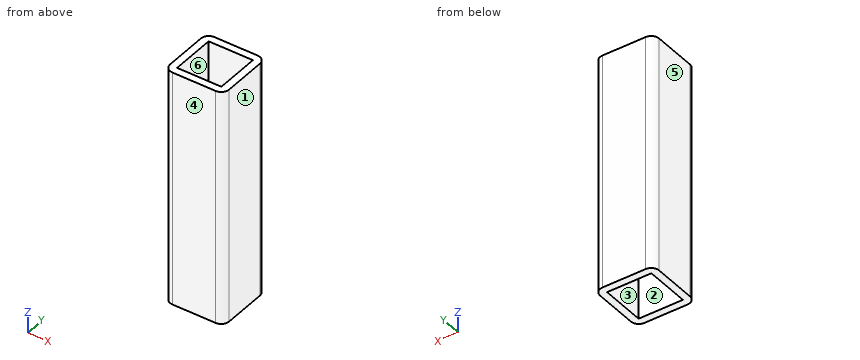
```python
from build123d import *

# Parameters (mm, degrees)
F0_W     = 38.1
F0_H     = 38.1
F0_W_2   = 28.575
F0_H_2   = 28.575
F1_DEPTH = 152.4
F2_R     = 5.08


with BuildPart() as f1:
    # F0 (on Top) → F1 (new body)
    with BuildSketch(Plane.XY):
        Rectangle(F0_W, F0_H)
        Rectangle(F0_W_2, F0_H_2, mode=Mode.SUBTRACT)
    extrude(amount=-F1_DEPTH)

    # F2
    f2_edges = [f1.edges().sort_by_distance(p)[0] for p in [
        (19.05, -19.05, -76.2),
        (19.05, 19.05, -76.2),
        (-19.05, -19.05, -76.2),
        (-19.05, 19.05, -76.2),
    ]]
    fillet(f2_edges, radius=F2_R)


solid = f1.part
```
Geometry check sheet. Reference: the model listing, model coordinates, mm. Face numbers are marked on the shaded views. A direction names the side the tool comes from. Round coordinates to 2 decimals unless told otherwise and drop trailing zeros. Order: outer loops, then holes, each group sorted by start corner. A loop starts at its lowest first (then second) coordinate and runs counter-clockwise, first axis right, second up. Notation, with made-up numbers: (19, 87.25) - (42, 87.25) arc R12 cw to (42, 103.25) - close; hole circle Ø10 at (-27.75, 86.25). An arc over 180 degrees is marked (long way). Use a Markdown table: item, result. Add a question column.
(1) Release check for a two-part mould opening along Y. For the marked faces 1, 2, 3 and 4 record: pulls with the +Y half, pulls with the -Y half, needs draft (parallel to the pull), parting line crosses it, or undercut.
(2) Material ranges on line 1 along X through (y, z) = (3.5, -39); line 2 along X through (y, z) = (14.5, -125.5), recorded low to high. Write a range as [from, to].
(3) Tool access check on the marked faces 5 and 6. Record the directions out of +Z, -Z, +X, -X, +Y, -Y that give a thin tool (end or side, any length) a straight path to the whole face; none if there is none.
(4) Sectioned sample at A-A, the plane x = -10. Enter the section's corners in (y, z).
(5) Sectioned sample at B-B, the plane z = -139.5. Enter the section's corners in (x, y), and give its area (3 significant figures).
Answers below:
| question | item | result |
|---|---|---|
| 1 | face 1 | needs draft |
| 1 | face 2 | undercut |
| 1 | face 3 | undercut |
| 1 | face 4 | pulls with the -Y half |
| 2 | line 1 | [-19.05, -14.29], [14.29, 19.05] |
| 2 | line 2 | [-19.02, 19.02] |
| 3 | face 5 | +Z, -Z, -X, +Y, -Y |
| 3 | face 6 | +Z, -Z |
| 4 | outline | (-19.05, -152.4) - (-14.29, -152.4) - (-14.29, 0) - (-19.05, 0) - close; (14.29, -152.4) - (19.05, -152.4) - (19.05, 0) - (14.29, 0) - close |
| 5 | outline | (-19.05, -13.97) arc R5.08 ccw to (-13.97, -19.05) - (13.97, -19.05) arc R5.08 ccw to (19.05, -13.97) - (19.05, 13.97) arc R5.08 ccw to (13.97, 19.05) - (-13.97, 19.05) arc R5.08 ccw to (-19.05, 13.97) - close; hole (-14.29, -14.29) - (14.29, -14.29) - (14.29, 14.29) - (-14.29, 14.29) - close |
| 5 | area | 613 mm² |
